```python
from build123d import *

# Parameters (mm, degrees)
SKETCH1_R           = 9
BOSS_EXTRUDE1_DEPTH = 1.5


with BuildPart() as part:
    # Sketch1 → Boss-Extrude1 (new, symmetric)
    with BuildSketch(Plane(origin=(0, 0, 0), x_dir=(1, 0, 0), z_dir=(0, 1, 0))):
        with BuildLine():
            Line((-8.613284174, -6.35), (-10.883410628, 2.104994632))
            ThreePointArc((-10.883410628, 2.104994632), (-8.533007766, 7.219663427), (-3.590944982, 9.91414778))
            Line((-3.590944982, 9.91414778), (3.443136374, 10.426476807))
            ThreePointArc((3.443136374, 10.426476807), (8.389040028, 7.361699028), (10.883410628, 2.104994632))
            Line((10.883410628, 2.104994632), (8.613284174, -6.35))
            ThreePointArc((8.613284174, -6.35), (0, -10.700988938), (-8.613284174, -6.35))
        make_face()
        with Locations(Location((0, 0, 0), (0, 0, 270))):
            Circle(SKETCH1_R, mode=Mode.SUBTRACT)
    extrude(amount=BOSS_EXTRUDE1_DEPTH, both=True)


solid = part.part
```
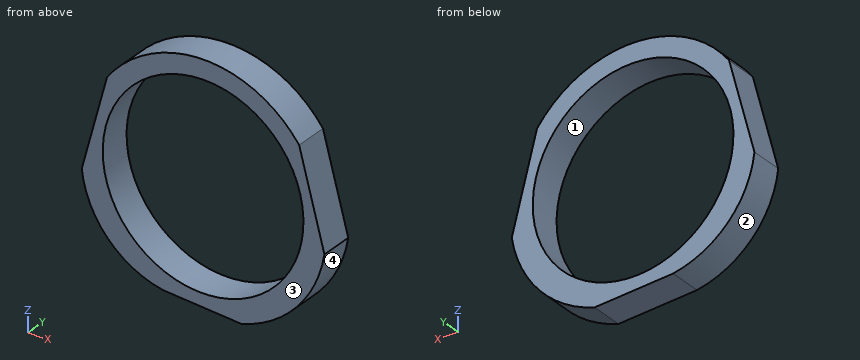
Part model, mm, in its own coordinate system. Face numbers are marked on the shaded views. Round coordinates to 2 decimals unless told otherwise and drop trailing zeros. Write each loop counter-clockwise with the first axis right and the second up, starting at its lowest first coordinate (ties: lowest second). Pieces come first, ordered by that corner, then holes. Notation, with made-up numbers: (3.5, -14.75) -> (7.5, -14.75) arc R19 cw to (7.5, -7.75) -> close; hole circle Ø5 at (67, 25.25). An arc over 180 degrees is marked (long way). Return JSON: item names as keys, results as strings. Group by question number.
Q1. Pin check, flat tips, straight feed: pin 1 (1 mm diameter, centred on y = 1, z = -7.5, fed in from +X); pin 2 (1 mm diameter, centred on y = 1, z = 0, fed in from +X); pin 3 (1 mm diameter, centred on x = 8.5, y = 0, fed in from +Z). Stop position of each tip, or through.
Q2. Mould opens along X. For the marked faces 1, 2, 3 and 4 say: pulls with the +X half, pulls with the -X half, needs draft (parallel to the pull), parting line crosses it, or undercut.
Q3. Saw through at A-A on z = -4.5. Write the cut outline in (x, y).
Q4. Saw through at B-B on x = 1.5. Write the cut outline in (y, z), plus the area to 3 significant figures.
Q5. Probe L1, parallel to X at y = -0.9, z = 5.75; L2, parallel to Z at x = 8, y = -0.5; L3, parallel to X at y = 0.7, z = 0. List the from-to ranges inside material, lowest first. Write a range as [from, to].
Answer:
{
 "1": {"pin 1": "x = 8.7", "pin 2": "x = 10.45", "pin 3": "z = 7.11"},
 "2": {"face 1": "undercut", "face 2": "pulls with the -X half", "face 3": "needs draft", "face 4": "pulls with the +X half"},
 "3": {"outline": "(-10.27, -1.5) -> (-7.79, -1.5) -> (-7.79, 1.5) -> (-10.27, 1.5) -> close; (7.79, -1.5) -> (10.2, -1.5) -> (10.2, 1.5) -> (7.79, 1.5) -> close"},
 "4": {"outline": "(-1.5, -10.28) -> (1.5, -10.28) -> (1.5, -8.87) -> (-1.5, -8.87) -> close; (-1.5, 8.87) -> (1.5, 8.87) -> (1.5, 10.6) -> (-1.5, 10.6) -> close", "area": "9.40 mm2"},
 "5": {"L1": "[-8.77, -6.92], [6.92, 8.77]", "L2": "[-7.77, -4.12], [4.12, 7.11]", "L3": "[-10.32, -9], [9, 10.32]"}
}
